Geometry check sheet. Reference: drawing and pictorial views, mm from the part's lowest x, y, z. Coordinates: 2 decimals unless noted, no trailing zeros. Loops run counter-clockwise (first coordinate to the right, second up) from the corner with the lowest first, then second, coordinate; pieces in that order, holes last. Notation, with made-up numbers: (46, 72.5) -> (81, 72.5) arc R24 ccw to (81, 85.5) -> close; hole circle Ø7 at (8, 29.5). An arc over 180 degrees is marked (long way). Answer as a JSON object with one key per item and string values. Group by question number.
Q1. Cross-section at B-B on z = 1.75. Give the number of separate pieces and of enclosed holes in the cut face, and give its area (3 significant figures).
Q2. Cross-section at C-C on y = 92. Record the boundary of the cut face in (x, z).
Q3. Scan lines: L1, parallel to Y at x = 99, z = 3.5; L2, parallel to X at y = 159, z = 1.5; L3, parallel to X at y = 209, z = 3.5. Record each from-to range of solid material in increasing order.
Q4. Cross-section at A-A on x = 142.5. Record the boundary of the cut face in (y, z), and give its area (3 significant figures).
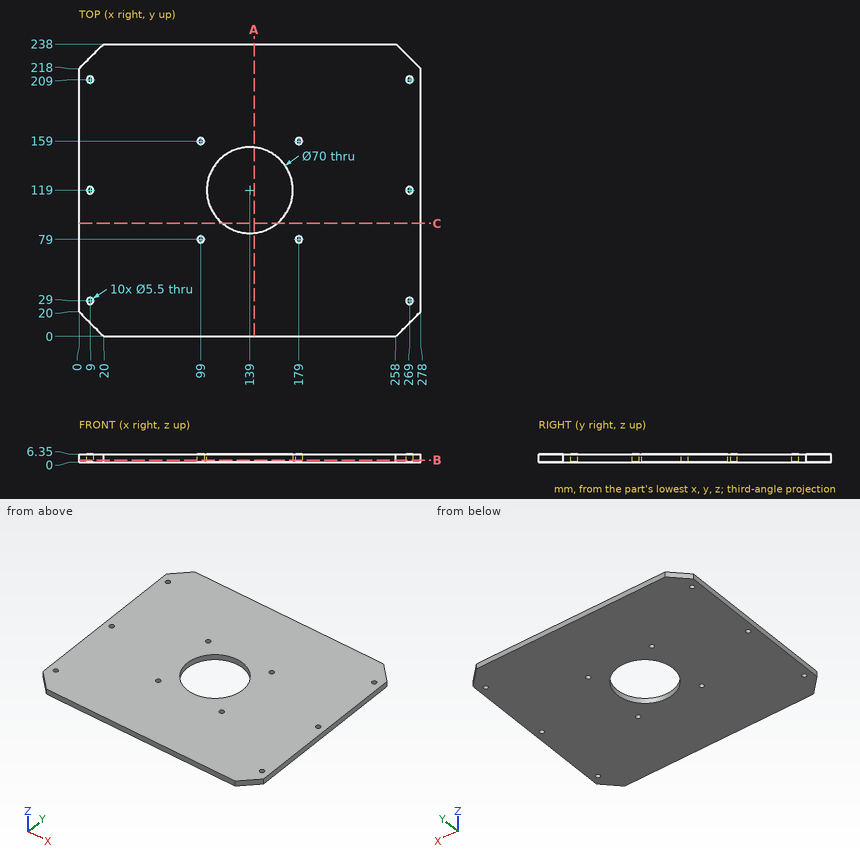
Computed values:
{
 "1": {"separate pieces": "1", "enclosed holes": "11", "area": "61,300 mm²"},
 "2": {"outline": "(0, 0) -> (116.73, 0) -> (116.73, 6.35) -> (0, 6.35) -> close; (161.27, 0) -> (278, 0) -> (278, 6.35) -> (161.27, 6.35) -> close"},
 "3": {"L1": "y = 0 to 76.25, 81.75 to 156.25, 161.75 to 238", "L2": "x = 0 to 96.25, 101.75 to 176.25, 181.75 to 278", "L3": "x = 0 to 6.25, 11.75 to 266.25, 271.75 to 278"},
 "4": {"outline": "(0, 0) -> (84.18, 0) -> (84.18, 6.35) -> (0, 6.35) -> close; (153.82, 0) -> (238, 0) -> (238, 6.35) -> (153.82, 6.35) -> close", "area": "1,070 mm²"}
}
